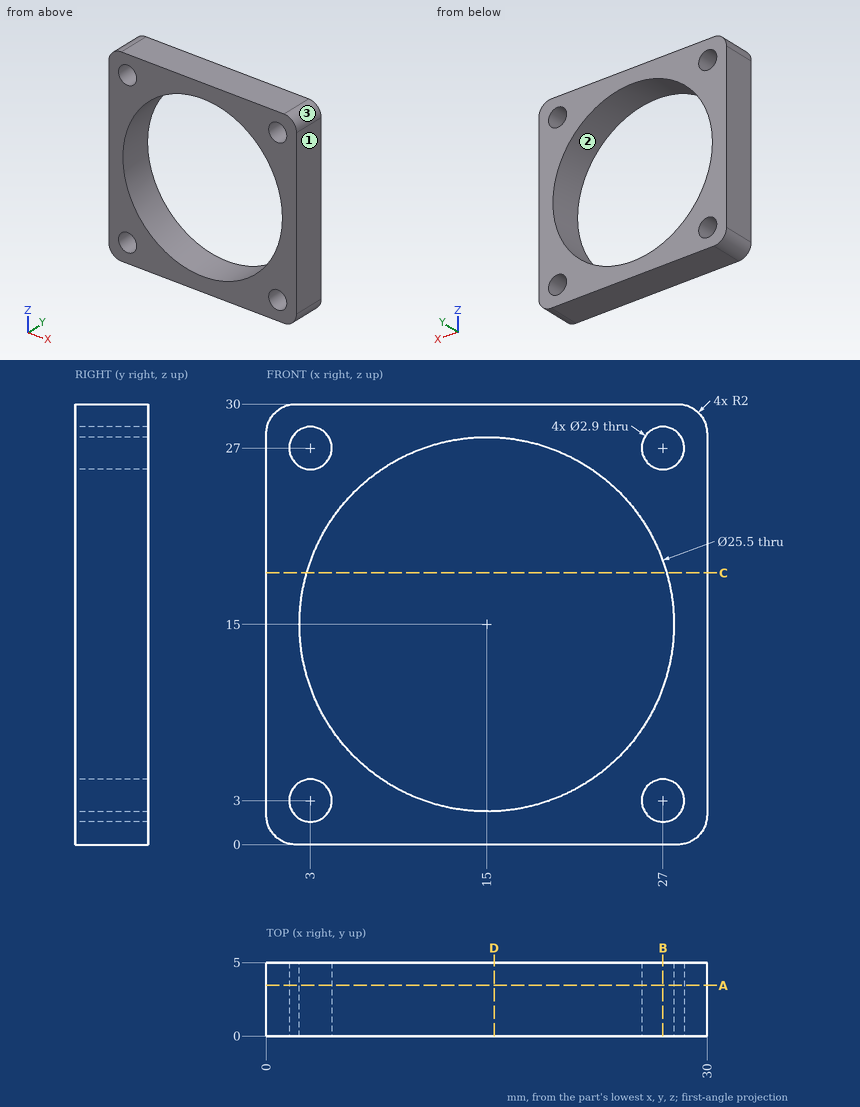
Input: dimensioned drawing with shaded views. Units: mm. Origin: part minimum x, y, z. Give positions to 0.01 mm unless a question says otherwise; leave off trailing zeros. Loops run counter-clockwise (first coordinate to the right, second up) from the corner with the lowest first, then second, coordinate; pieces in that order, holes last. Notation, with made-up numbers: (71.25, -34.75) -> (99.25, -34.75) arc R23 ccw to (99.25, -24.75) -> close; hole circle Ø3 at (59.25, 14.5). An arc over 180 degrees is marked (long way). Use a Markdown table: item, result.
Q1. Pull-direction query (Z, two-part tool) for the marked faces 1, 2 and 3; classes: pulls with the +Z half, pulls with the -Z half, needs draft (parallel to the pull), parting line crosses it, or undercut.
Entries:
| item | result |
|---|---|
| face 1 | needs draft |
| face 2 | undercut |
| face 3 | pulls with the +Z half |
Q2. Section query A-A, the plane y = 3.45. Return the cut outline in (x, z), plus the area to 3 significant figures.
Entries:
| item | result |
|---|---|
| outline | (0, 2) arc R2 ccw to (2, 0) -> (28, 0) arc R2 ccw to (30, 2) -> (30, 28) arc R2 ccw to (28, 30) -> (2, 30) arc R2 ccw to (0, 28) -> close; hole circle Ø2.9 at (3, 3); hole circle Ø2.9 at (3, 27); hole circle Ø25.5 at (15, 15); hole circle Ø2.9 at (27, 3); hole circle Ø2.9 at (27, 27) |
| area | 359 mm² |
Q3. Ray query, probe 1 along Z at (x, y) = (15, 2); probe 2 along X at (y, z) = (1.8, 28); probe 3 along Z at (x, y) = (20.25, 4). Return the intervals inside material, ascending. Write a range as from..to.
Entries:
| item | result |
|---|---|
| probe 1 | z = 0..2.25, 27.75..30 |
| probe 2 | x = 0..1.95, 4.05..25.95, 28.05..30 |
| probe 3 | z = 0..3.38, 26.62..30 |
Q4. Section query C-C, the plane z = 18.5. Return the cut outline in (x, y), plus the area to 3 significant figures.
Entries:
| item | result |
|---|---|
| outline | (0, 0) -> (2.74, 0) -> (2.74, 5) -> (0, 5) -> close; (27.26, 0) -> (30, 0) -> (30, 5) -> (27.26, 5) -> close |
| area | 27.4 mm² |
Q5. Section query D-D, the plane x = 15.5. Return the cut outline in (y, z).
Entries:
| item | result |
|---|---|
| outline | (0, 0) -> (5, 0) -> (5, 2.26) -> (0, 2.26) -> close; (0, 27.74) -> (5, 27.74) -> (5, 30) -> (0, 30) -> close |
Q6. Section query B-B, the plane x = 27. Return the cut outline in (y, z), plus the area to 3 significant figures.
Entries:
| item | result |
|---|---|
| outline | (0, 0) -> (5, 0) -> (5, 1.55) -> (0, 1.55) -> close; (0, 4.45) -> (5, 4.45) -> (5, 10.69) -> (0, 10.69) -> close; (0, 19.31) -> (5, 19.31) -> (5, 25.55) -> (0, 25.55) -> close; (0, 28.45) -> (5, 28.45) -> (5, 30) -> (0, 30) -> close |
| area | 77.9 mm² |
